Model file for the job. Use its own axes, mm. Face numbers are marked on the shaded views. Round coordinates to 2 decimals unless told otherwise and drop trailing zeros. Loops run counter-clockwise (first coordinate to the right, second up) from the corner with the lowest first, then second, coordinate; pieces in that order, holes last. Notation, with made-up numbers: (4, 61) - (28, 61) arc R21 cw to (28, 87) - close; hole circle Ø4 at (81, -23.5). An arc over 180 degrees is marked (long way). Answer as a JSON object with one key per item and string values.
from build123d import *

# Parameters (mm, degrees)
SKETCH1_R               = 17
SKETCH1_R_2             = 0.49999999999999895
SKETCH1_R_3             = 6
SKETCH1_R_4             = 0.4999999999999985
SKETCH1_R_5             = 0.49999999999999967
SKETCH1_R_6             = 0.5000000000000008
BOSS_EXTRUDE1_DEPTH     = 1.5
SKETCH7_W               = 0.5
SKETCH7_H               = 0.5
CUT_EXTRUDE1_DEPTH      = 25.794152536434876
CUT_EXTRUDE1_DEPTH_BACK = 25.794152536434876
CUT_EXTRUDE2_DEPTH      = 25.92990172463582
CUT_EXTRUDE2_DEPTH_BACK = 25.92990172463582
SKETCH5_R               = 0.5000000000000009
SKETCH5_R_2             = 0.48729793970449836
FILLET1_R               = 0.5
CHAMFER1_SIZE           = 1
FILLET2_R               = 1


with BuildPart() as part:
    # Sketch1 → Boss-Extrude1 (new, symmetric)
    with BuildSketch(Plane.XY):
        Circle(SKETCH1_R)
        with Locations((9.600000000000001, 0)):
            Circle(SKETCH1_R_2, mode=Mode.SUBTRACT)
        Circle(SKETCH1_R_3, mode=Mode.SUBTRACT)
        with Locations((-3.352e-14, -9.600000000000001)):
            Circle(SKETCH1_R_4, mode=Mode.SUBTRACT)
        with Locations((-9.600000000000001, 6.704e-14)):
            Circle(SKETCH1_R_5, mode=Mode.SUBTRACT)
        with Locations((1.0055e-13, 9.600000000000001)):
            Circle(SKETCH1_R_6, mode=Mode.SUBTRACT)
    extrude(amount=BOSS_EXTRUDE1_DEPTH, both=True)

    # Sketch2 → Cut-Revolve1 (revolve, cut)
    with BuildSketch(Plane(origin=(0, 0, 0), x_dir=(1, 0, 0), z_dir=(0, 1, 0)), mode=Mode.PRIVATE) as cut_revolve1_sk:
        with BuildLine():
            Line((-16.5, -0.49999999999999956), (-16.5, 0.49999999999999956))
            ThreePointArc((-16.5, 0.49999999999999956), (-16.646446609406727, 0.8535533905932733), (-17, 1))
            Line((-17, 1), (-17, -1))
            ThreePointArc((-17, -1), (-16.646446609406727, -0.8535533905932733), (-16.5, -0.49999999999999956))
        make_face()
    revolve(cut_revolve1_sk.sketch.rotate(Axis((0, 0, 0), (0, 0, -1)), 180), axis=Axis((0, 0, 0), (0, 0, -1)), mode=Mode.SUBTRACT)

    # Sketch7 → Revolve1 (revolve)
    with BuildSketch(Plane(origin=(0, 0, 0), x_dir=(1, 0, 0), z_dir=(0, 1, 0))):
        with Locations((17.25, 1.25)):
            Rectangle(SKETCH7_W, SKETCH7_H)
        with Locations((17.25, -1.25)):
            Rectangle(SKETCH7_W, SKETCH7_H)
    revolve(axis=Axis((0, 0, 0), (0, 0, -1)))

    # Sketch4 → Cut-Extrude1 (cut, two sides: drawn at the far end of the back side and taken through both)
    with BuildSketch(Plane.XY.offset(-CUT_EXTRUDE1_DEPTH_BACK)):
        Polygon((-3.3089929101566358, 18.76623133261556), (0, 0), (18.766231332615533, -3.308992910156828), (18.766231332615533, -21.784688156780618), (-24.932091474912426, -21.784688156780618), (-24.93209147491243, 18.76623133261556), align=None)
    extrude(amount=CUT_EXTRUDE1_DEPTH + CUT_EXTRUDE1_DEPTH_BACK, mode=Mode.SUBTRACT)

    # Sketch5 → Cut-Extrude2 (cut, two sides: drawn at the far end of the back side and taken through both)
    with BuildSketch(Plane.XY.offset(1.5).offset(-CUT_EXTRUDE2_DEPTH_BACK)):
        with Locations((-2.439480379102094, 13.834980723316052)):
            Circle(SKETCH5_R)
        with Locations((-0.37984462011943565, 14.021287153916445)):
            Circle(SKETCH5_R_2)
    extrude(amount=CUT_EXTRUDE2_DEPTH + CUT_EXTRUDE2_DEPTH_BACK, mode=Mode.SUBTRACT)

    # Fillet1
    fillet1_edges = [part.edges().sort_by_distance(p)[0] for p in [
        (4.242640687119308, 4.242640687119264, 1.5),
        (4.242640687119308, 4.242640687119264, -1.5),
    ]]
    fillet(fillet1_edges, radius=FILLET1_R)

    # Chamfer1
    chamfer1_edges = [part.edges().sort_by_distance(p)[0] for p in [
        (9.100000000000003, 6e-17, 1.5),
        (-0.49999999999990025, 9.600000000000001, 1.5),
    ]]
    chamfer(chamfer1_edges, length=CHAMFER1_SIZE)

    # Fillet2
    fillet2_edges = [part.edges().sort_by_distance(p)[0] for p in [
        (17.23413567771362, -3.0388431091714043, 1.25),
        (-3.0388431091712285, 17.23413567771365, -1.25),
    ]]
    fillet(fillet2_edges, radius=FILLET2_R - 0.0001)  # a hair under: the kernel refuses the full size


solid = part.part
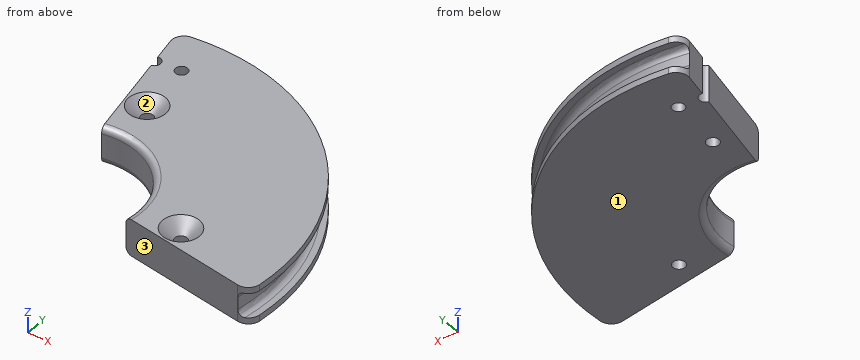
1) Slice it at C-C on z = -0.2. Count the separate pieces of the cut face and the enclosed holes in it, then the cut area to 3 significant figures.
Values follow:
{"separate pieces": "1", "enclosed holes": "3", "area": "224 mm²"}
2) Two-plate mould, pull along X, no slides. Class the marked faces 1, 2 and 3: pulls with the +X half, pulls with the -X half, needs draft (parallel to the pull), parting line crosses it, or undercut.
Values follow:
{"face 1": "needs draft", "face 2": "undercut", "face 3": "pulls with the -X half"}
3) Slice it at B-B on z = -1.25. List the corners of the cut face in (x, y), then the cut area to 3 significant figures.
Values follow:
{"outline": "(-2.86, 16.22) - (-2.53, 14.33) arc R0.5 cw to (-2.35, 13.34) - (-1.05, 5.97) arc R6.07 cw to (5.97, -1.05) - (16.22, -2.86) arc R1 ccw to (17.39, -1.99) arc R17.5 ccw to (-1.99, 17.39) arc R1 ccw to start; hole circle Ø0.97 at (-0.38, 14.02); hole circle Ø1 at (0, 9.6); hole circle Ø1 at (9.6, 0)", "area": "255 mm²"}
4) Probe probe 1 along Y at (x, z) = (-0.5, 1.35); probe 2 along Y at (x, z) = (0, -0.3); probe 3 along Y at (x, z) = (10.5, 1.05). List the from-to ranges inside material, lowest first.
Values follow:
{"probe 1": "6.12 to 8.35, 10.85 to 13.55, 14.49 to 17.49", "probe 2": "6 to 9.1, 10.1 to 13.72, 14.33 to 16.5", "probe 3": "-1.85 to -0.54, 0.54 to 14"}
5) Slice it at A-A on y = 0. List the corners of the cut face in (x, z).
Values follow:
{"outline": "(6, -1) arc R0.5 ccw to (6.5, -1.5) - (9.1, -1.5) - (9.1, 0.5) - (8.1, 1.5) - (6.5, 1.5) arc R0.5 ccw to (6, 1) - close; (10.1, -1.5) - (17.5, -1.5) - (17.5, -1) - (17, -1) arc R0.5 cw to (16.5, -0.5) - (16.5, 0.5) arc R0.5 cw to (17, 1) - (17.5, 1) - (17.5, 1.5) - (11.1, 1.5) - (10.1, 0.5) - close"}
